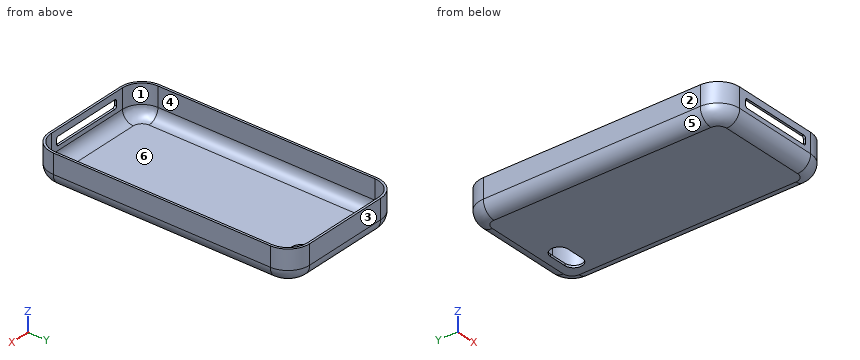
from build123d import *

# Parameters (mm, degrees)
F0_W     = 76.2
F0_H     = 152.4
F1_DEPTH = 19.05
F2_R     = 12.7
F3_R     = 7.62
F4_T     = -1.27
F6_DEPTH = 25.4
F8_DEPTH = 25.4


with BuildPart() as f1:
    # F0 (on Top) → F1 (new body)
    with BuildSketch(Plane.XY):
        with Locations((-12.107471, 8.866039)):
            Rectangle(F0_W, F0_H)
    extrude(amount=F1_DEPTH)

    # F2
    f2_edges = [f1.edges().sort_by_distance(p)[0] for p in [
        (25.992529, 85.066039, 9.525),
        (25.992529, -67.333961, 9.525),
        (-50.207471, 85.066039, 9.525),
        (-50.207471, -67.333961, 9.525),
    ]]
    fillet(f2_edges, radius=F2_R)

    # F3
    f3_edges = [f1.edges().sort_by_distance(p)[0] for p in [
        (-50.207471, 8.866039, 0),
        (-46.487727, 81.346295, 0),
        (-46.487727, -63.614217, 0),
        (-12.107471, 85.066039, 0),
        (-12.107471, -67.333961, 0),
        (22.272785, 81.346295, 0),
        (22.272785, -63.614217, 0),
        (25.992529, 8.866039, 0),
    ]]
    fillet(f3_edges, radius=F3_R)

    # F4
    f4_openings = [f1.faces().sort_by_distance(p)[0] for p in [
        (-12.107471, 8.866039, 19.05),
    ]]
    offset(amount=F4_T, openings=f4_openings)

    # F5 (on face) → F6 (cut)
    with BuildSketch(Plane(origin=(0, 0, 0), x_dir=(1, 0, 0), z_dir=(0, 0, -1))):
        with BuildLine():
            Line((-1.987378, -72.366039), (8.199227, -72.366039))
            ThreePointArc((8.199227, -72.366039), (13.292529, -67.272736), (8.199227, -62.179434))
            Line((8.199227, -62.179434), (-1.987378, -62.179434))
            ThreePointArc((-1.987378, -62.179434), (-7.08068, -67.272736), (-1.987378, -72.366039))
        make_face()
    extrude(amount=-F6_DEPTH, mode=Mode.SUBTRACT)

    # F7 (on face) → F8 (cut)
    with BuildSketch(Plane.XZ.offset(67.333961)):
        with BuildLine():
            Line((8.356589, 15.24), (-32.028437, 15.24))
            ThreePointArc((-32.028437, 15.24), (-32.926462, 14.868026), (-33.298437, 13.97))
            Line((-33.298437, 13.97), (-33.298437, 11.43))
            ThreePointArc((-33.298437, 11.43), (-32.926462, 10.531974), (-32.028437, 10.16))
            Line((-32.028437, 10.16), (8.356589, 10.16))
            ThreePointArc((8.356589, 10.16), (9.254614, 10.531974), (9.626589, 11.43))
            Line((9.626589, 11.43), (9.626589, 13.97))
            ThreePointArc((9.626589, 13.97), (9.254614, 14.868026), (8.356589, 15.24))
        make_face()
    extrude(amount=-F8_DEPTH, mode=Mode.SUBTRACT)


solid = f1.part
Source: CAD feature listing. Evaluate the final solid. Frame: model axes, mm. Face numbers are marked on the shaded views. A direction names the side the tool comes from. Give positions to 0.01 mm unless a question says otherwise; leave off trailing zeros. Write each loop counter-clockwise with the first axis right and the second up, starting at its lowest first coordinate (ties: lowest second). Pieces come first, ordered by that corner, then holes. Notation, with made-up numbers: M 1.25,71.5 L 47.25,71.5 A19 cw 47.25,95.5 Z; hole C 12.5,60 d10. An arc over 180 degrees is marked long. Return JSON: item names as keys, results as strings. Group by question number.
1) Material intervals for line 1 along X through (y, z) = (-11, 10); line 2 along Y through (x, z) = (-37.5, 8); line 3 along Z through (x, y) = (-14.5, 69), sorted ascending. Write a range as [from, to].
2) Cut plane A-A, the plane x = 6.5. Output: boundary loops of the cut face in (y, z), plus the area to 3 significant figures.
3) Pin query (flat end, axial travel): P1, Ø1.5, axis at x = -36, y = -1.5, coming from the +Z side; P2, Ø2, axis at x = -22.5, z = 11.5, coming from the -Y side; P3, Ø0.6, axis at x = 4.5, z = 0.5, coming from the +Y side; P4, Ø1.5, axis at x = 2, z = 7, coming from the -Y side. Return the tip coordinate at first contact, or that it passes through.
4) Set-up query: the marked faces 5 and 6. Return all of +Z, -Z, +X, -X, +Y, -Y with unobstructed straight access to the full face (end or side cutting, diameter ignored); none if empty.
5) Cut plane B-B, the plane x = -23. Output: boundary loops of the cut face in (y, z), plus the area to 3 significant figures.
6) Cut plane D-D, the plane z = 17. Output: boundary loops of the cut face in (x, y).
7) Pull-direction query (X, two-part tool) for the marked faces 1, 2, 3 and 4; classes: pulls with the +X half, pulls with the -X half, needs draft (parallel to the pull), parting line crosses it, or undercut.
8) Cut plane C-C, the plane y = 6. Output: boundary loops of the cut face in (x, z).
Recorded:
{
 "1": {"line 1": "x = [-50.21, -48.94], [24.72, 25.99]", "line 2": "y = [-67.33, -66.06], [83.8, 85.07]", "line 3": "z = [0, 1.27]"},
 "2": {"outline": "M -67.33,7.62 A7.62 ccw -59.71,0 L 62.18,0 L 62.18,1.27 L -59.71,1.27 A6.35 cw -66.06,7.62 L -66.06,10.16 L -67.33,10.16 Z; M -67.33,15.24 L -66.06,15.24 L -66.06,19.05 L -67.33,19.05 Z; M 72.37,0 L 77.45,0 A7.62 ccw 85.07,7.62 L 85.07,19.05 L 83.8,19.05 L 83.8,7.62 A6.35 cw 77.45,1.27 L 72.37,1.27 Z", "area": "212 mm²"},
 "3": {"P1": "stops at z = 1.27", "P2": "stops at y = 83.8", "P3": "stops at y = 80.84", "P4": "stops at y = -67.33"},
 "4": {"face 5": "-Z, -X, +Y, -Y", "face 6": "+Z"},
 "5": {"outline": "M -67.33,7.62 A7.62 ccw -59.71,0 L 77.45,0 A7.62 ccw 85.07,7.62 L 85.07,19.05 L 83.8,19.05 L 83.8,7.62 A6.35 cw 77.45,1.27 L -59.71,1.27 A6.35 cw -66.06,7.62 L -66.06,10.16 L -67.33,10.16 Z; M -67.33,15.24 L -66.06,15.24 L -66.06,19.05 L -67.33,19.05 Z", "area": "225 mm²"},
 "6": {"outline": "M -50.21,-54.63 A12.7 ccw -37.51,-67.33 L 13.29,-67.33 A12.7 ccw 25.99,-54.63 L 25.99,72.37 A12.7 ccw 13.29,85.07 L -37.51,85.07 A12.7 ccw -50.21,72.37 Z; hole M -48.94,-54.63 A11.43 ccw -37.51,-66.06 L 13.29,-66.06 A11.43 ccw 24.72,-54.63 L 24.72,72.37 A11.43 ccw 13.29,83.8 L -37.51,83.8 A11.43 ccw -48.94,72.37 Z"},
 "7": {"face 1": "undercut", "face 2": "pulls with the -X half", "face 3": "needs draft", "face 4": "undercut"},
 "8": {"outline": "M -50.21,7.62 A7.62 ccw -42.59,0 L 18.37,0 A7.62 ccw 25.99,7.62 L 25.99,19.05 L 24.72,19.05 L 24.72,7.62 A6.35 cw 18.37,1.27 L -42.59,1.27 A6.35 cw -48.94,7.62 L -48.94,19.05 L -50.21,19.05 Z"}
}
